Autodesk Inventor part; units mm, degrees
ref_plane "Work Plane1" through (20.3835, 0, -31.4198) normal (1, 0, 0) x (0, 1, 0)
ref_plane "Work Plane2" through (0, 0, -31.4198) normal (0, 0, -1) x (-1, 0, 0)
ref_plane "Work Plane3" through (20.3835, 0, -31.4198) normal (-1, 0, 0) x (0, 0, 1)
sketch "Sketch1" plane through (0, 0, 0) normal (0, 0, 1) x (1, 0, 0)
  circle A0 centre (0, 0) radius 20.3835
  dimension "d0" = 40.767
extrude "Extrusion1" add sketch "Sketch1" against normal blind 31.4198
sketch "Sketch2" plane through (0, 0, -31.4198) normal (0, 0, -1) x (-1, 0, 0)
  circle A0 centre (0, 0) radius 20.3835
  line L0 (-20.3835, 0) -> (-20.3835, 24.6473)
ref_plane "Work Plane1" through (20.3835, 0, -31.4198) normal (1, 0, 0) x (0, 1, 0)
sketch "Sketch3" plane through (20.3835, 0, -31.4198) normal (1, 0, 0) x (0, 1, 0)
  line L0 (-20.3835, 0) -> (20.3835, 0)
  line L1 (0, 0) -> (0, -20.3835)
  circle A0 centre (0, -20.3835) radius 20.3835
  point P0 (0, 31.4198)
  dimension "d4" = 20.3835
extrude "Extrusion2" add sketch "Sketch3" along normal blind 31.4198
sketch "Sketch4" plane through (0, 0, 0) normal (0, 0, 1) x (1, 0, 0)
  circle A0 centre (0, 0) radius 16.7767
  dimension "d7" = 33.5534
sketch "Sketch5" plane through (51.8033, 0, -51.8033) normal (1, 0, 0) x (0, 0, -1)
  circle A0 centre (0, 0) radius 16.7767
  point P0 (-51.8033, 0)
  dimension "d8" = 33.5534
ref_plane "Work Plane2" through (0, 0, -31.4198) normal (0, 0, -1) x (-1, 0, 0)
ref_plane "Work Plane3" through (20.3835, 0, -31.4198) normal (-1, 0, 0) x (0, 0, 1)
revolve "Revolution1" add sketch "Sketch2" angle 90 about axis through (20.3835, 0, -31.4198) along (0, -1, 0)
extrude "Extrusion3" cut sketch "Sketch4" against normal blind 31.75
sketch "Sketch6" plane through (0, 0, -31.4198) normal (0, 0, -1) x (-1, 0, 0)
  circle A0 centre (0, 0) radius 12.7
  line L0 (-20.3835, -28.5369) -> (-20.3835, 28.5369)
  dimension "d14" = 25.4
revolve "Revolution2" cut sketch "Sketch6" angle 90 about axis through (20.3835, 0, -31.4198) along (0, -1, 0)
extrude "Extrusion4" cut sketch "Sketch5" against normal blind 31.75
properties part number "90 Elbow 1 Inch"
Source: CAD feature listing. Evaluate the final solid. Frame: model axes, mm. A direction names the side the tool comes from. Give positions to 0.01 mm unless a question says otherwise; leave off trailing zeros. Order: outer loops, then holes, each group sorted by start corner. A loop starts at its lowest first (then second) coordinate and runs counter-clockwise, first axis right, second up.
(1) Section query B-B (x = 36.5). Return the cut outline in (y, z), plus the area to 3 significant figures.
(2) Access query for faces 4 (the face through (19.442, 6.123, -15.49)), 5 (the face through (-17, -3, 0)), 6 (the face through (35.9, -4.4, -31.9)). Directions: +Z, -Z, +X, -X, +Y, -Y. A direction counts if a zero-diameter tool reaches every point of the face in a straight line with its end or side. Return the directions, or none.
(3) Pull-direction query (X, two-part tool) for faces 1 (the face through (-3, 13, -31.75)), 2 (the face through (36.151, 0.738, -35.043)), 3 (the face through (51.803, -17, -55)); classes: +X half, -X half, draft (parallel to the pull), parting line (faces both ways), or undercut.
(4) Material intervals for line 1 along Y through (x, z) = (0, -13); line 2 along X through (y, z) = (0.5, -6); line 3 along Y through (x, z) = (35, -37.5), sorted ascending.
(5) Contact query for flat-ended pins moving along their axis: P1, Ø6, axis at y = -5.5, z = -63, coming from the -X side; P2, Ø4, axis at x = 27, z = -49.5, coming from the -Y side; P3, Ø1.5, axis at x = 1.5, z = -21.5, coming from the +Y side. Output: stop coordinate, or through.
(6) Section query A-A (z = -26). Return the cut outline in (x, y), plus the area to 3 significant figures.
Outcome:
1. outline: circle Ø40.77 at (0, -51.8); hole circle Ø33.55 at (0, -51.8)
1. area: 421 mm2
2. face 4: +Z
2. face 5: +Z, +X, -X, +Y, -Y
2. face 6: +X
3. face 1: undercut
3. face 2: draft
3. face 3: +X half
4. line 1: y = -20.38 to -16.78, 16.78 to 20.38
4. line 2: x = -20.38 to -16.77, 16.77 to 20.38
4. line 3: y = -14.52 to -8.77, 8.77 to 14.52
5. P1: stops at x = -7.81
5. P2: stops at y = -20.38
5. P3: stops at y = 20.37
6. outline: circle Ø40.77 at (0, 0); hole circle Ø33.55 at (0, 0)
6. area: 421 mm2
